The drawing under review shows one solid part. Ordinate dimensions are in mm from its lowest x, y, z. Round coordinates to 2 decimals unless told otherwise and drop trailing zeros. Loops run counter-clockwise (first coordinate to the right, second up) from the corner with the lowest first, then second, coordinate; pieces in that order, holes last. Notation, with made-up numbers: (-18.75, -15.75) - (1.25, -15.75) arc R19 ccw to (1.25, -10.75) - close; hole circle Ø5 at (84, 0.5). An arc over 180 degrees is marked (long way). Answer as CSV lines item,"result".
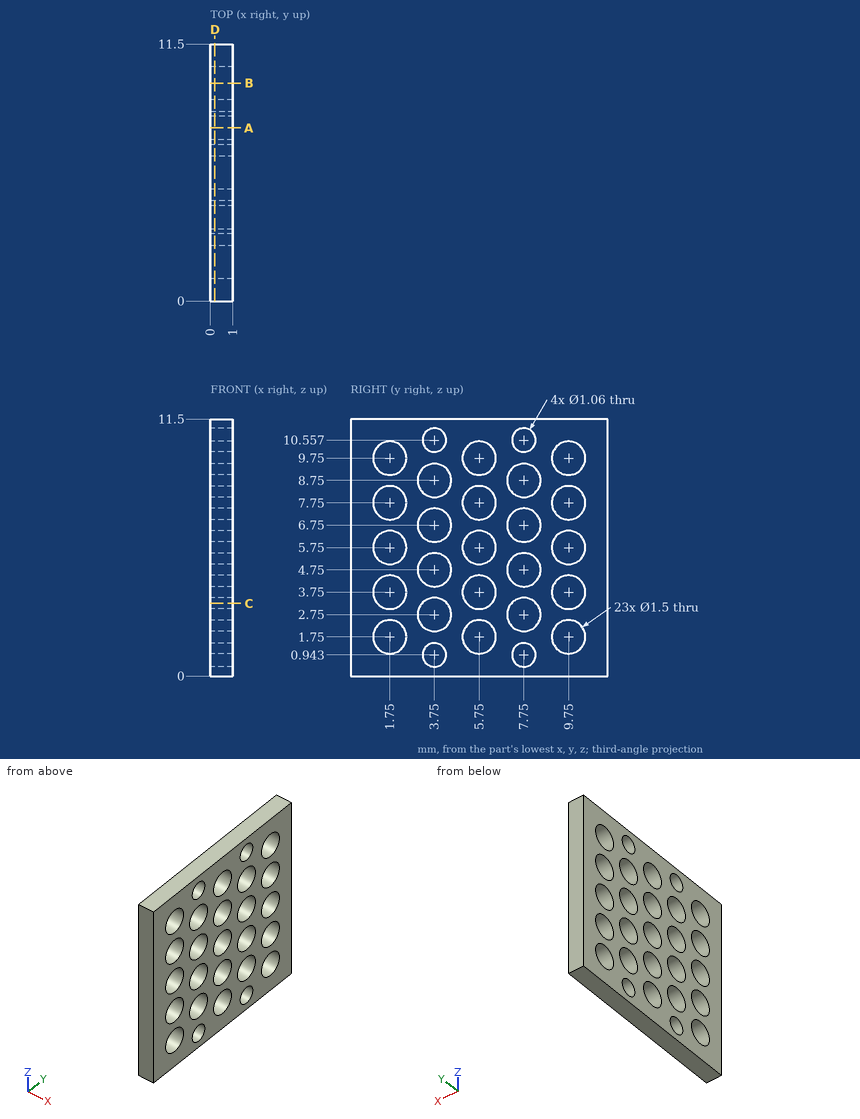
1. Wall thickness on probe 1 along Z at (x, y) = (0.85, 9.5); probe 2 along Y at (x, z) = (0.6, 5.25): over which ranges is each line inside the solid? List them lowest first.
Numbers:
probe 1,"z = 0 to 1.04, 2.46 to 3.04, 4.46 to 5.04, 6.46 to 7.04, 8.46 to 9.04, 10.46 to 11.5"
probe 2,"y = 0 to 1.19, 2.31 to 3.19, 4.31 to 5.19, 6.31 to 7.19, 8.31 to 9.19, 10.31 to 11.5"
2. Take a section at C-C (z = 3.25). State the section outline as (x, y) points.
Numbers:
outline,"(0, 0) - (1, 0) - (1, 1.19) - (0, 1.19) - close; (0, 2.31) - (1, 2.31) - (1, 3.19) - (0, 3.19) - close; (0, 4.31) - (1, 4.31) - (1, 5.19) - (0, 5.19) - close; (0, 6.31) - (1, 6.31) - (1, 7.19) - (0, 7.19) - close; (0, 8.31) - (1, 8.31) - (1, 9.19) - (0, 9.19) - close; (0, 10.31) - (1, 10.31) - (1, 11.5) - (0, 11.5) - close"
3. Take a section at B-B (y = 9.75). State the section outline as (x, z) points.
Numbers:
outline,"(0, 0) - (1, 0) - (1, 1) - (0, 1) - close; (0, 2.5) - (1, 2.5) - (1, 3) - (0, 3) - close; (0, 4.5) - (1, 4.5) - (1, 5) - (0, 5) - close; (0, 6.5) - (1, 6.5) - (1, 7) - (0, 7) - close; (0, 8.5) - (1, 8.5) - (1, 9) - (0, 9) - close; (0, 10.5) - (1, 10.5) - (1, 11.5) - (0, 11.5) - close"
4. Take a section at A-A (y = 7.75). State the section outline as (x, z) points.
Numbers:
outline,"(0, 0) - (1, 0) - (1, 0.41) - (0, 0.41) - close; (0, 1.47) - (1, 1.47) - (1, 2) - (0, 2) - close; (0, 3.5) - (1, 3.5) - (1, 4) - (0, 4) - close; (0, 5.5) - (1, 5.5) - (1, 6) - (0, 6) - close; (0, 7.5) - (1, 7.5) - (1, 8) - (0, 8) - close; (0, 9.5) - (1, 9.5) - (1, 10.03) - (0, 10.03) - close; (0, 11.09) - (1, 11.09) - (1, 11.5) - (0, 11.5) - close"
5. Take a section at D-D (x = 0.2). State how many separate pieces and enclosed holes the cut face has.
Numbers:
separate pieces,"1"
enclosed holes,"27"
6. Clearance check with flat-ended pins moving along their axes: pin 1 (1.2 mm diameter, centred on y = 1.75, z = 7.75, fed in from +X); pin 2 (4 mm diameter, centred on y = 3.5, z = 8.5, fed in from +X). State where each tip first meets the part, or that it passes through.
Numbers:
pin 1,"passes through"
pin 2,"stops at x = 1"
